from build123d import *

# Parameters (mm, degrees)
F0_W     = 101.6
F0_H     = 152.4
F0_W_2   = 76.2
F0_H_2   = 127
F1_DEPTH = 63.5
F2_DEPTH = 12.7


with BuildPart() as f1:
    # F0 (on Front) → F1 (new body)
    with BuildSketch(Plane.XZ):
        Rectangle(F0_W, F0_H)
        with Locations((0, -1.875399)):
            Rectangle(F0_W_2, F0_H_2, mode=Mode.SUBTRACT)
    extrude(amount=F1_DEPTH)

    # F0 (on Front) → F2 (join)
    with BuildSketch(Plane.XZ):
        with Locations((0, -1.875399)):
            Rectangle(F0_W_2, F0_H_2)
    extrude(amount=F2_DEPTH)


solid = f1.part
Could you check a few things on this model? Use its own coordinates, in mm. A direction names the side the tool comes from. Coordinates: 2 decimals unless noted, no trailing zeros. Order: outer loops, then holes, each group sorted by start corner. A loop starts at its lowest first (then second) coordinate and runs counter-clockwise, first axis right, second up. Notation, with made-up numbers: (-13.5, -29) -> (7.5, -29) arc R21 ccw to (7.5, 8) -> close; hole circle Ø7 at (20.25, 16). An arc over 180 degrees is marked (long way). One line per item, written item: value. Start each with the question number.
1) Imagine slicing it at B-B on x = 7. List the corners of the cut face in (y, z) for me, plus the area to 3 significant figures.
2) I'm going to push a flat-ended pin straight in: pin 1 (5 mm diameter, centred on x = 20, z = -38, fed in from -Y). Where does the tip first touch, or does it pass through?
3) Imagine slicing it at C-C on z = 31. List the corners of the cut face in (x, y) for me, plus the area to 3 significant figures.
4) Which directions (+Z, -Z, +X, -X, +Y, -Y) give clear straight access to the entire face, cutting with the end or side of a thin tool? Please do faces 5 (the flat face through (-1, -31, 76.2)), 6 (the flat face through (-1, -12.7, -1)).
5) We'd pull the mould along Z, two halves only. Please class faces 1 (the flat face through (-38.1, -38, -3)), 2 (the flat face through (44, -63.5, 1)), 3 (the flat face through (-1, -38, 61.625)), 4 (the flat face through (-1, -31, -76.2)): +Z half, -Z half, draft (parallel to the pull), parting line (faces both ways), or undercut.
6) If I drill on L1, parallel to X at y = -56, z = 3; L2, parallel to Z at x = 6, y = -16; L3, parallel to Y at x = 4.5, z = 50, over which ranges is the centre line in solid material (lowest first)? Write a range as [from, to].
7) Imagine slicing it at A-A on y = -26. List the corners of the cut face in (x, z) for me, plus the area to 3 significant figures.
Answer list:
1. outline: (-63.5, -76.2) -> (0, -76.2) -> (0, 76.2) -> (-63.5, 76.2) -> (-63.5, 61.62) -> (-12.7, 61.62) -> (-12.7, -65.38) -> (-63.5, -65.38) -> close
1. area: 3,230 mm2
2. pin 1: stops at y = -12.7
3. outline: (-50.8, -63.5) -> (-38.1, -63.5) -> (-38.1, -12.7) -> (38.1, -12.7) -> (38.1, -63.5) -> (50.8, -63.5) -> (50.8, 0) -> (-50.8, 0) -> close
3. area: 2,580 mm2
4. face 5: +Z, +X, -X, +Y, -Y
4. face 6: -Y
5. face 1: undercut
5. face 2: draft
5. face 3: undercut
5. face 4: -Z half
6. L1: x = [-50.8, -38.1], [38.1, 50.8]
6. L2: z = [-76.2, -65.38], [61.62, 76.2]
6. L3: y = [-12.7, 0]
7. outline: (-50.8, -76.2) -> (50.8, -76.2) -> (50.8, 76.2) -> (-50.8, 76.2) -> close; hole (-38.1, -65.38) -> (38.1, -65.38) -> (38.1, 61.62) -> (-38.1, 61.62) -> close
7. area: 5,810 mm2
